Geometry: final body of the model. Coordinates: model frame, mm. A direction names the side the tool comes from. Give positions to 0.01 mm unless a question says otherwise; leave off trailing zeros. Write each loop counter-clockwise with the first axis right and the second up, starting at its lowest first coordinate (ties: lowest second). Pieces come first, ordered by that corner, then holes. Notation, with made-up numbers: (89, 47) -> (111, 47) arc R23 cw to (111, 59) -> close; hole circle Ø4 at (65, -5). An arc over 180 degrees is marked (long way). Answer as a JSON object with one key per item and string values.
from build123d import *

# Parameters (mm, degrees)
SKETCH_1_R      = 2.4
EXTRUDE_1_DEPTH = 6


with BuildPart() as part:
    # 草图1 → 凸台-拉伸1 (new body)
    # profile 1 of 2: a face of its own
    with BuildSketch(Plane(origin=(0, 0, 0), x_dir=(1, 0, 0), z_dir=(0, 1, 0))):
        Polygon((35.26180856, 66.984800923), (-9.73819144, 66.984800923), (-9.73819144, 36.984800923), (-9.73819144, 29.984800923), (-1.73819144, 29.984800923), (-1.73819144, 45.484800923), (27.26180856, 45.484800923), (27.26180856, -17.515199077), (-1.73819144, -17.515199077), (-1.73819144, -2.015199077), (-9.73819144, -2.015199077), (-9.73819144, -9.015199077), (-9.73819144, -39.015199077), (35.26180856, -39.015199077), align=None)
        with Locations(Location((31.26180856, -7.015199077, 0), (0, 0, 270))):
            Circle(SKETCH_1_R, mode=Mode.SUBTRACT)
        with Locations(Location((-5.73819144, 34.984800923, 0), (0, 0, 270))):
            Circle(SKETCH_1_R, mode=Mode.SUBTRACT)
    # profile 2 of 2: a face of its own
    with BuildSketch(Plane(origin=(0, 0, 0), x_dir=(1, 0, 0), z_dir=(0, 1, 0))):
        Polygon((-9.73819144, 29.984800923), (-9.73819144, 36.984800923), (-19.73819144, 36.984800923), (-19.73819144, -9.015199077), (-9.73819144, -9.015199077), (-9.73819144, -2.015199077), (-11.73819144, -2.015199077), (-11.73819144, 29.984800923), align=None)
    extrude(amount=EXTRUDE_1_DEPTH)


solid = part.part
Q1. Cut plane D-D (z = -59). Return the cut outline in (x, y).
Values:
{"outline": "(-9.74, 0) -> (35.26, 0) -> (35.26, 6) -> (-9.74, 6) -> close"}
Q2. Cut plane A-A (z = 10.5). Return the cut outline in (x, y).
Values:
{"outline": "(-9.74, 0) -> (-1.74, 0) -> (-1.74, 6) -> (-9.74, 6) -> close; (27.26, 0) -> (35.26, 0) -> (35.26, 6) -> (27.26, 6) -> close"}
Q3. Cut plane C-C (y = 2). Return the cut outline in (x, z), and give its area (3 significant figures).
Values:
{"outline": "(-19.74, -36.98) -> (-9.74, -36.98) -> (-9.74, -66.98) -> (35.26, -66.98) -> (35.26, 39.02) -> (-9.74, 39.02) -> (-9.74, 9.02) -> (-19.74, 9.02) -> close; hole (-11.74, -29.98) -> (-1.74, -29.98) -> (-1.74, -45.48) -> (27.26, -45.48) -> (27.26, 17.52) -> (-1.74, 17.52) -> (-1.74, 2.02) -> (-11.74, 2.02) -> close; hole circle Ø4.8 at (-5.74, -34.98); hole circle Ø4.8 at (31.26, 7.02)", "area": "3,050 mm²"}
Q4. Material intervals for L1, parallel to X at y = 0.6, z = -41; L2, parallel to Z at x = -6, y = 5.5; L3, parallel to X at y = 1.9, z = -0.5, sorted ascending. Write a range as from..to.
Values:
{"L1": "-9.74..-1.74, 27.26..35.26", "L2": "-66.98..-37.37, -32.6..-29.98, 2.02..39.02", "L3": "-19.74..-11.74, 27.26..35.26"}
Q5. First-contact query: P1, Ø3, axis at x = -16.5, y = 3, coming from the +Z side; P2, Ø3, axis at y = 2.5, z = 27.5, coming from the -X side; P3, Ø1, axis at x = -12, y = 3.5, coming from the -Z side; P4, Ø4.5, axis at x = 31.26, z = 7.02, coming from the +Y side. Flat tips, straight axial feed; report the tip coordinate or a pass-through.
Values:
{"P1": "z = 9.02", "P2": "x = -9.74", "P3": "z = -36.98", "P4": "through"}
Q6. Cut plane B-B (x = 12.5). Return the cut outline in (y, z).
Values:
{"outline": "(0, -66.98) -> (6, -66.98) -> (6, -45.48) -> (0, -45.48) -> close; (0, 17.52) -> (6, 17.52) -> (6, 39.02) -> (0, 39.02) -> close"}
Q7. Mould query, pull axis Z, two halves, no side actions, for faces 6 (the flat face through (-19.738, 3, -14)), 7 (the flat face through (13, 3, -45.485)), 8 (the flat face through (13, 3, -66.985)). Classes: pulls with the +Z half, pulls with the -Z half, needs draft (parallel to the pull), parting line crosses it, or undercut.
Values:
{"face 6": "needs draft", "face 7": "undercut", "face 8": "pulls with the -Z half"}
Q8. Set-up query: faces 1 (the flat face through (-15, 3, 9.015)), 2 (the flat face through (-9.738, 3, -52)), 3 (the flat face through (-11.738, 3, -14)), 4 (the flat face through (12, 3, 39.015)), 5 (the flat face through (32, 6, -15)). Return all of +Z, -Z, +X, -X, +Y, -Y with unobstructed straight access to the full face (end or side cutting, diameter ignored); none if empty.
Values:
{"face 1": "+Z, -X, +Y, -Y", "face 2": "-Z, -X, +Y, -Y", "face 3": "+Y, -Y", "face 4": "+Z, +X, -X, +Y, -Y", "face 5": "+Z, -Z, +X, -X, +Y"}
